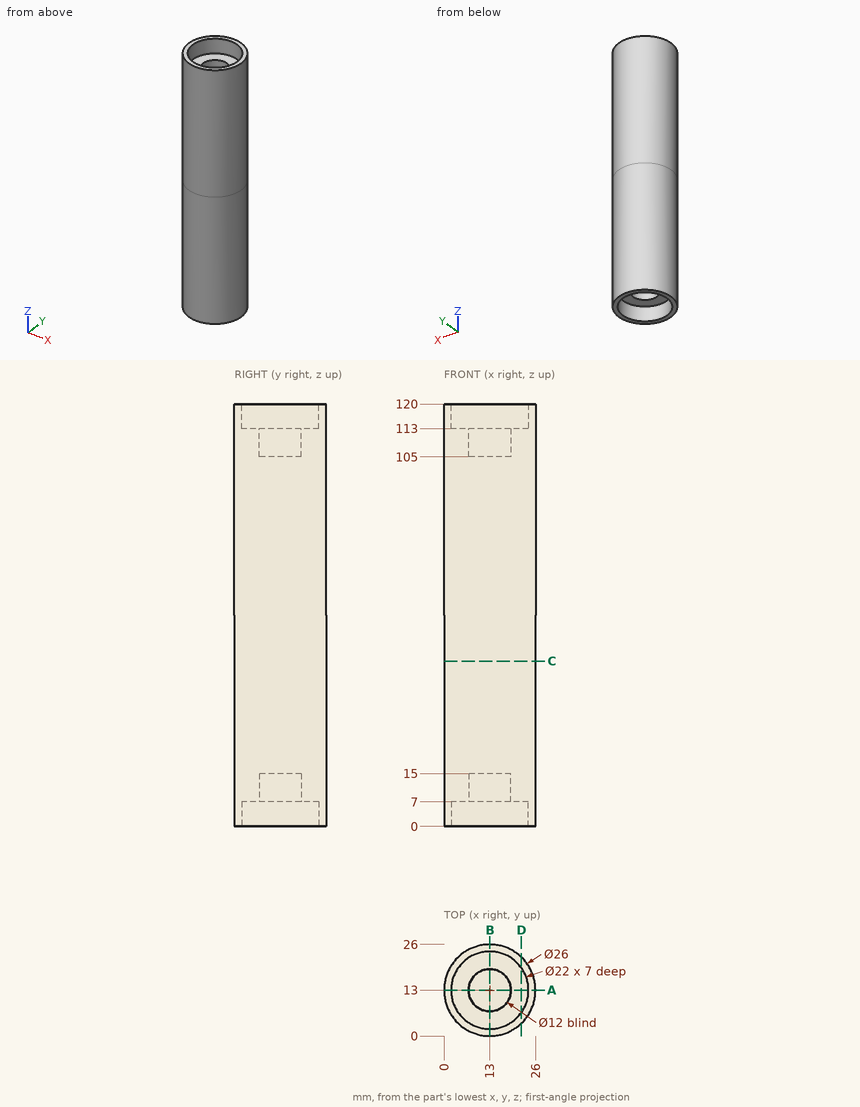
Check sheet for the drawn part. Datum: minimum x, y, z corner. Units: mm. Round coordinates to 2 decimals unless told otherwise and drop trailing zeros. Write each loop counter-clockwise with the first axis right and the second up, starting at its lowest first coordinate (ties: lowest second). Pieces come first, ordered by that corner, then holes. Notation, with made-up numbers: (-33, 75) -> (5, 75) arc R28 cw to (5, 110) -> close; hole circle Ø5 at (32, 58). An arc over 180 degrees is marked (long way). One line per item, written item: value. Start each with the question number.
(1) Scan lines: line 1 (Y direction, x = 13, z = 9); line 2 (Y direction, x = 13, z = 5); line 3 (Z direction, x = 19.5, y = 6.5). Record each from-to range of solid material in increasing order. Write a range as [from, to].
(2) Cross-section at C-C, the plane z = 47. Record the cut outline in (x, y).
(3) Cross-section at A-A, the plane y = 13. Record the cut outline in (x, z).
(4) Go/stop test with flat-tipped pins: pin 1 Ø2 at (y, z) = (10.5, 89.5) entering from +X; pin 2 Ø3 at (y, z) = (9.5, 87) entering from +X; pin 3 Ø5 at (x, z) = (5, 73.5) entering from -Y. Record where each tip stops, or that it passes through.
(5) Cross-section at D-D, the plane x = 22. Record the cut outline in (y, z), and give its area (3 significant figures).
Answer:
1. line 1: [0, 7], [19, 26]
1. line 2: [0, 2], [24, 26]
1. line 3: [7, 113]
2. outline: circle Ø26 at (13, 13)
3. outline: (0, 0) -> (2, 0) -> (2, 7) -> (7, 7) -> (7, 15) -> (19, 15) -> (19, 7) -> (24, 7) -> (24, 0) -> (26, 0) -> (26, 120) -> (24, 120) -> (24, 113) -> (19, 113) -> (19, 105) -> (7, 105) -> (7, 113) -> (2, 113) -> (2, 120) -> (0, 120) -> close
4. pin 1: x = 25.91
4. pin 2: x = 25.85
4. pin 3: y = 1.22
5. outline: (3.62, 0) -> (6.68, 0) -> (6.68, 7) -> (19.32, 7) -> (19.32, 0) -> (22.38, 0) -> (22.38, 120) -> (19.32, 120) -> (19.32, 113) -> (6.68, 113) -> (6.68, 120) -> (3.62, 120) -> close
5. area: 2,070 mm²
